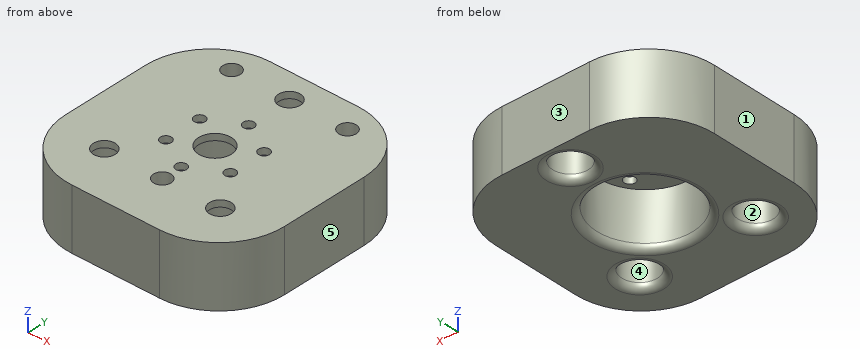
from build123d import *

# Parameters (mm, degrees)
SKETCH1_W           = 100
SKETCH1_H           = 100
SKETCH1_R           = 2.5
SKETCH1_R_2         = 7.5
SKETCH1_R_3         = 5
BOSS_EXTRUDE1_DEPTH = 3
SKETCH2_W           = 100
SKETCH2_H           = 100
SKETCH2_R           = 8.1
SKETCH2_R_2         = 22
BOSS_EXTRUDE2_DEPTH = 25
FILLET2_R           = 3
FILLET3_R           = 3
SKETCH3_R           = 4
CUT_EXTRUDE1_DEPTH  = 25
FILLET4_R           = 30


with BuildPart() as part:
    # Sketch1 → Boss-Extrude1 (new body)
    with BuildSketch(Plane.XY):
        Rectangle(SKETCH1_W, SKETCH1_H)
        with Locations((-14.722431864, 8.5)):
            Circle(SKETCH1_R, mode=Mode.SUBTRACT)
        with Locations((-14.722431864, -8.5)):
            Circle(SKETCH1_R, mode=Mode.SUBTRACT)
        with Locations((0, -17)):
            Circle(SKETCH1_R, mode=Mode.SUBTRACT)
        with Locations((14.722431864, -8.5)):
            Circle(SKETCH1_R, mode=Mode.SUBTRACT)
        with Locations((14.722431864, 8.5)):
            Circle(SKETCH1_R, mode=Mode.SUBTRACT)
        with Locations((0, 17)):
            Circle(SKETCH1_R, mode=Mode.SUBTRACT)
        Circle(SKETCH1_R_2, mode=Mode.SUBTRACT)
        with Locations((0, 37.5)):
            Circle(SKETCH1_R_3, mode=Mode.SUBTRACT)
        with Locations((-26.516504294, -26.516504295)):
            Circle(SKETCH1_R_3, mode=Mode.SUBTRACT)
        with Locations((26.516504294, -26.516504295)):
            Circle(SKETCH1_R_3, mode=Mode.SUBTRACT)
    extrude(amount=BOSS_EXTRUDE1_DEPTH)

    # Sketch2 → Boss-Extrude2 (add)
    with BuildSketch(Plane(origin=(0, 0, 0), x_dir=(-1, 0, 0), z_dir=(0, 0, -1))):
        Rectangle(SKETCH2_W, SKETCH2_H)
        with Locations(Location((-26.516504294, -26.516504294, 0), (0, 0, 180))):
            Circle(SKETCH2_R, mode=Mode.SUBTRACT)
        with Locations(Location((26.516504294, -26.516504294, 0), (0, 0, 180))):
            Circle(SKETCH2_R, mode=Mode.SUBTRACT)
        with Locations(Location((0, 37.5, 0), (0, 0, 180))):
            Circle(SKETCH2_R, mode=Mode.SUBTRACT)
        with Locations(Location((0, 0, 0), (0, 0, 180))):
            Circle(SKETCH2_R_2, mode=Mode.SUBTRACT)
    extrude(amount=BOSS_EXTRUDE2_DEPTH)

    # Fillet2
    fillet2_edges = [part.edges().sort_by_distance(p)[0] for p in [
        (-8.1, 37.5, -25),
        (-34.616504294, -26.516504294, -25),
        (18.416504295, -26.516504294, -25),
    ]]
    fillet(fillet2_edges, radius=FILLET2_R)

    # Fillet3
    fillet3_edges = [part.edges().sort_by_distance(p)[0] for p in [
        (-22, 0, -25),
    ]]
    fillet(fillet3_edges, radius=FILLET3_R)

    # Sketch3 → Cut-Extrude1 (cut)
    with BuildSketch(Plane.XY.offset(3)):
        with Locations((26.516504294, 37.5)):
            Circle(SKETCH3_R)
        with Locations((-26.516504294, 37.5)):
            Circle(SKETCH3_R)
        with Locations((0, -26.516504294)):
            Circle(SKETCH3_R)
    extrude(amount=-CUT_EXTRUDE1_DEPTH, mode=Mode.SUBTRACT)

    # Fillet4
    fillet4_edges = [part.edges().sort_by_distance(p)[0] for p in [
        (-50, 50, -11),
        (50, 50, -11),
        (50, -50, -11),
        (-50, -50, -11),
    ]]
    fillet(fillet4_edges, radius=FILLET4_R)


solid = part.part
Design review of the part built by this model. Coordinates are the model's own, in mm. Face numbers are marked on the shaded views. A direction names the side the tool comes from. Give positions to 0.01 mm unless a question says otherwise; leave off trailing zeros. Order: outer loops, then holes, each group sorted by start corner. A loop starts at its lowest first (then second) coordinate and runs counter-clockwise, first axis right, second up. Notation, with made-up numbers: (-5, -25) - (24, -25) arc R27 cw to (24, 7) - close; hole circle Ø9 at (27, 32). An arc over 180 degrees is marked (long way). Write item = value, one per line. Start each with the question number.
Q1. We need section A-A on z = -13. State the section outline as (x, y) points, plus the area to 3 significant figures.
Q2. Mouldability with a two-part tool opening along Y and no side actions: class the marked faces 1, 2 and 3 as released by +Y, released by -Y, zero draft, split by the parting line, or undercut.
Q3. To check wall thickness, follow L1, parallel to Y at x = 0, z = -12.5; L2, parallel to Y at x = -12, z = -20.5; L3, parallel to Y at x = -30, z = -5.25. State the ranges of each line that lie inside material, in increasing order. Write a range as from..to.
Q4. Tool access review of the marked faces 4 and 5: name each direction out of +Z, -Z, +X, -X, +Y, -Y from which nothing blocks a thin tool from reaching the whole face with its end or side.
Q5. Clearance check with flat-ended pins moving along their axes: pin 1 Ø4 at (x, y) = (-1.5, -27) entering from +Z; pin 2 Ø14.5 at (x, y) = (26.52, -26.52) entering from -Z; pin 3 Ø4.5 at (x, y) = (14.72, -8.5) entering from +Z; pin 4 Ø18.5 at (x, y) = (-26.52, -26.52) entering from -Z. State where each tip first meets the part, or that it passes through.
Working result:
q1.outline = (-50, -20) arc R30 ccw to (-20, -50) - (20, -50) arc R30 ccw to (50, -20) - (50, 20) arc R30 ccw to (20, 50) - (-20, 50) arc R30 ccw to (-50, 20) - close; hole circle Ø16.2 at (-26.52, -26.52); hole circle Ø8 at (-26.52, 37.5); hole circle Ø44 at (0, 0); hole circle Ø16.2 at (0, 37.5); hole circle Ø8 at (0, -26.52); hole circle Ø16.2 at (26.52, -26.52); hole circle Ø8 at (26.52, 37.5)
q1.area = 6,940 mm²
q2.face_1 = zero draft
q2.face_2 = undercut
q2.face_3 = released by +Y
q3.L1 = -50..-30.52, -22.52..-22, 22..29.4, 45.6..50
q3.L2 = -50..-18.44, 18.44..50
q3.L3 = -48.28..-33.83, -19.2..35.53, 39.47..48.28
q4.face_4 = -Z
q4.face_5 = +Z, -Z, +X, +Y, -Y
q5.pin_1 = -22
q5.pin_2 = 0
q5.pin_3 = through
q5.pin_4 = -24.37
